The model under review builds one solid part; all positions refer to its coordinate system, in mm. A direction names the side the tool comes from. Coordinates: 2 decimals unless noted, no trailing zeros. Order: outer loops, then holes, each group sorted by start corner. A loop starts at its lowest first (then second) coordinate and runs counter-clockwise, first axis right, second up.
```python
from build123d import *

# Parameters (mm, degrees)
CROQUIS2_W                   = 20
CROQUIS2_H                   = 20
SALIENTE_EXTRUIR1_DEPTH      = 50
CROQUIS3_W                   = 20
CROQUIS3_H                   = 20
SALIENTE_EXTRUIR2_DEPTH      = 51
SALIENTE_EXTRUIR4_DEPTH      = 60
SALIENTE_EXTRUIR4_DEPTH_BACK = 20
CROQUIS7_W                   = 30
CROQUIS7_H                   = 10
CROQUIS8_R                   = 1.4
CORTAR_EXTRUIR2_DEPTH        = 60
CROQUIS9_R                   = 12.395
CORTAR_EXTRUIR3_DEPTH        = 5


with BuildPart() as part:
    # Croquis2 → Saliente-Extruir1 (new body)
    with BuildSketch(Plane.XY):
        Rectangle(CROQUIS2_W, CROQUIS2_H)
    extrude(amount=SALIENTE_EXTRUIR1_DEPTH)

    # Croquis3 → Saliente-Extruir2 (add)
    with BuildSketch(Plane(origin=(0, 10, 0), x_dir=(1, 0, 0), z_dir=(0, 1, 0))):
        with Locations((0, -40)):
            Rectangle(CROQUIS3_W, CROQUIS3_H)
    extrude(amount=SALIENTE_EXTRUIR2_DEPTH)

    # Croquis7 → Saliente-Extruir4 (add, two sides: drawn at the far end of the back side and taken through both)
    with BuildSketch(Plane(origin=(0, 0, 30), x_dir=(-1, 0, 0), z_dir=(0, 0, -1)).offset(-SALIENTE_EXTRUIR4_DEPTH_BACK)):
        with Locations((0, 60)):
            Rectangle(CROQUIS7_W, CROQUIS7_H)
    extrude(amount=SALIENTE_EXTRUIR4_DEPTH + SALIENTE_EXTRUIR4_DEPTH_BACK)

    # Croquis8 → Cortar-Extruir2 (cut)
    with BuildSketch(Plane(origin=(0, 65, 0), x_dir=(1, 0, 0), z_dir=(0, 1, 0))):
        with Locations(Location((0, 5, 0), (0, 0, 270))):
            Circle(CROQUIS8_R)
    extrude(amount=-CORTAR_EXTRUIR2_DEPTH, mode=Mode.SUBTRACT)

    # Croquis9 → Cortar-Extruir3 (cut)
    with BuildSketch(Plane(origin=(0, 65, 0), x_dir=(1, 0, 0), z_dir=(0, 1, 0))):
        with Locations(Location((0, 5, 0), (0, 0, 270))):
            Circle(CROQUIS9_R)
    extrude(amount=-CORTAR_EXTRUIR3_DEPTH, mode=Mode.SUBTRACT)


solid = part.part
```
(1) Wall thickness on probe 1 along X at (y, z) = (57.7, -5); probe 2 along Y at (x, z) = (-7.25, 22.5); probe 3 along Y at (x, z) = (-10.75, 32.5): over which ranges is each line inside the solid? List them lowest first.
A:
probe 1: x = -15 to -1.4, 1.4 to 15
probe 2: y = -10 to 10, 55 to 65
probe 3: y = 55 to 65
(2) We need section A-A, the plane z = 24. Write out the cut boundary in (x, y).
A:
outline: (-15, 55) - (15, 55) - (15, 65) - (-15, 65) - close; (-10, -10) - (10, -10) - (10, 10) - (-10, 10) - close
(3) Draft analysis for pull direction Y (two halves, no side actions). For faces 6 (the face through (-3, 60, -5)), 7 (the face through (-15, 60, 11)), 8 (the face through (0, 55, 2)), state which applies: released by +Y, released by -Y, zero draft, split by the parting line, or undercut.
A:
face 6: released by +Y
face 7: zero draft
face 8: undercut
(4) For pin 1 Ø16 at (x, y) = (0.5, -4.5) entering from -Z; pin 2 Ø6 at (y, z) = (1.5, 34.5) entering from -X; pin 3 Ø12 at (x, y) = (9.5, 17.5) entering from -Z, all flat-tipped, find the tip position at first contact; note any pin that passes through.
A:
pin 1: stops at z = 0
pin 2: stops at x = -10
pin 3: stops at z = 30
(5) Machinability: for faces 1 (the face through (3.723, 62.535, 6.823)), 2 (the face through (-10, 15, 31)), 3 (the face through (10, 15, 31)), 4 (the face through (0, 32, 30)), 5 (the face through (0, 0, 0)), which of the approach directions +Z, -Z, +X, -X, +Y, -Y give a long, thin tool a straight path to every point of the face, cutting with its end or side? Answer none if there is none.
A:
face 1: +Y
face 2: +Z, -Z, -X, -Y
face 3: +Z, -Z, +X, -Y
face 4: -Z, +X, -X
face 5: -Z, +X, -X, -Y
(6) We need section D-D, the plane y = 4.5. Write out the cut boundary in (x, z).
A:
outline: (-10, 0) - (10, 0) - (10, 50) - (-10, 50) - close
(7) We need section C-C, the plane z = -5. Write out the cut boundary in (x, y) (3 decimals), and give its area (3 significant figures).
A:
outline: (-15, 55) - (-1.4, 55) - (-1.4, 60) - (-12.395, 60) - (-12.395, 65) - (-15, 65) - close; (1.4, 55) - (15, 55) - (15, 65) - (12.395, 65) - (12.395, 60) - (1.4, 60) - close
area: 162 mm2
(8) We need section B-B, the plane x = 0. Write out the cut boundary in (y, z) (3 decimals).
A:
outline: (-10, 0) - (10, 0) - (10, 30) - (55, 30) - (55, -3.6) - (60, -3.6) - (60, 7.395) - (65, 7.395) - (65, 50) - (-10, 50) - close; (55, -30) - (65, -30) - (65, -17.395) - (60, -17.395) - (60, -6.4) - (55, -6.4) - close
